Check sheet for the modelled part. Datum: model origin and axes. Units: mm. A direction names the side the tool comes from. Give positions to 0.01 mm unless a question says otherwise; leave off trailing zeros. Order: outer loops, then holes, each group sorted by start corner. A loop starts at its lowest first (then second) coordinate and runs counter-clockwise, first axis right, second up.
```python
from build123d import *

# Parameters (mm, degrees)
SKETCH1_R           = 5
BOSS_EXTRUDE1_DEPTH = 20
SKETCH2_R           = 0.75
CUT_EXTRUDE1_DEPTH  = 15


with BuildPart() as part:
    # Sketch1 → Boss-Extrude1 (new body)
    with BuildSketch(Plane(origin=(0, 0, 0), x_dir=(1, 0, 0), z_dir=(0, 1, 0))):
        with Locations(Location((0, 0, 0), (0, 0, 270))):
            Circle(SKETCH1_R)
        with BuildLine():
            Line((-3.464101615, 2), (-2.598076211, 1.5))
            ThreePointArc((-2.598076211, 1.5), (0, 3), (2.598076211, 1.5))
            Line((2.598076211, 1.5), (3.464101615, 2))
            ThreePointArc((3.464101615, 2), (0, 4), (-3.464101615, 2))
        make_face(mode=Mode.SUBTRACT)
    extrude(amount=BOSS_EXTRUDE1_DEPTH)

    # Sketch2 → Cut-Extrude1 (cut)
    with BuildSketch(Plane.XZ):
        with Locations(Location((0, 0, 0), (0, 0, 270))):
            Circle(SKETCH2_R)
    extrude(amount=-CUT_EXTRUDE1_DEPTH, mode=Mode.SUBTRACT)


solid = part.part
```
(1) Sectioned sample at B-B (z = 0). Enter the section's corners in (x, y).
(2) Sectioned sample at D-D (y = 3.5). Enter the section's corners in (x, z), plus the area to 3 significant figures.
(3) Thickness scan on L1, parallel to X at y = 8.25, z = -2.25; L2, parallel to X at y = 5, z = 0; L3, parallel to Z at x = -1.75, y = 12.75. Record the ranges inside material, lowest first.
(4) Release check for a two-part mould opening along X. For faces 1 (the face through (3.03, 9.86, -1.75)), 2 (the face through (-4.88, 9.86, -1.08)), 3 (the face through (0, 0, 1)) record: released by +X, released by -X, zero draft, split by the parting line, or undercut.
(5) Sectioned sample at A-A (x = 0). Enter the section's corners in (y, z).
(6) Sectioned sample at C-C (z = -3.5). Enter the section's corners in (x, y).
(7) Tool access check on faces 4 (the face through (0, 20, 0)), 5 (the face through (-3.037, 9.86, -1.754)), 6 (the face through (0.225, 7.395, -0.715)). Record the directions out of +Z, -Z, +X, -X, +Y, -Y that give a thin tool (end or side, any length) a straight path to the whole face; none if there is none.
(8) Go/stop test with flat-tipped pins: P1, Ø1, axis at y = 17, z = 2.5, coming from the -X side; P2, Ø5, axis at y = 12.5, z = 2, coming from the +X side; P3, Ø2, axis at y = 16.5, z = -3.5, coming from the -X side. Record where each tip stops, or that it passes through.
Values follow:
1. outline: (-5, 0) - (-0.75, 0) - (-0.75, 15) - (0.75, 15) - (0.75, 0) - (5, 0) - (5, 20) - (-5, 20) - close
2. outline: circle Ø10 at (0, 0); hole (-3.46, -2) arc R4 ccw to (3.46, -2) - (2.6, -1.5) arc R3 cw to (-2.6, -1.5) - close; hole circle Ø1.5 at (0, 0)
2. area: 69.4 mm2
3. L1: x = -4.47 to -3.31, -1.98 to 1.98, 3.31 to 4.47
3. L2: x = -5 to -0.75, 0.75 to 5
3. L3: z = -4.68 to -3.6, -2.44 to 4.68
4. face 1: undercut
4. face 2: split by the parting line
4. face 3: zero draft
5. outline: (0, -5) - (20, -5) - (20, -4) - (0, -4) - close; (0, -3) - (20, -3) - (20, 5) - (0, 5) - (0, 0.75) - (15, 0.75) - (15, -0.75) - (0, -0.75) - close
6. outline: (-3.57, 0) - (-1.94, 0) - (-1.94, 20) - (-3.57, 20) - close; (1.94, 0) - (3.57, 0) - (3.57, 20) - (1.94, 20) - close
7. face 4: +Z, -Z, +X, -X, +Y
7. face 5: +Y, -Y
7. face 6: -Y
8. P1: stops at x = -4.58
8. P2: stops at x = 5
8. P3: stops at x = -4.33
